Model file for the job. Use its own axes, mm. A direction names the side the tool comes from. Give positions to 0.01 mm unless a question says otherwise; leave off trailing zeros. Loops run counter-clockwise (first coordinate to the right, second up) from the corner with the lowest first, then second, coordinate; pieces in that order, holes last. Notation, with made-up numbers: (69.5, -7.5) -> (89.5, -7.5) arc R31 cw to (89.5, 25.5) -> close; hole circle Ø9 at (37.25, 19). An arc over 180 degrees is marked (long way). Use CSV: the item, a comma, the result in double quotes. Start each with the question number.
(1) Cut at B-B on y = 0.5. Write the cut outline in (x, z), then the cut area to 3 significant figures.
(2) Pull direction Y, two halves, no side cores. Call faces 6 (the cylindrical face through (4, 24, 0)), 7 (the cylindrical face through (-8.028, -9.157, -0.111)), 8 (the cylindrical face through (-0.084, 12.926, -0.238)), 9 (the flat face through (-3, 8, -10)): pulls with the +Y half, pulls with the -Y half, needs draft (parallel to the pull), parting line crosses it, or undercut.
(3) Flat gauge pins, fed straight in: pin 1 (1.3 mm diameter, centred on y = 14, z = 0, fed in from -X); pin 2 (1.5 mm diameter, centred on y = 8, z = 5, fed in from +X); pin 3 (6 mm diameter, centred on y = 14.5, z = 0, fed in from -X); pin 4 (1.5 mm diameter, centred on x = 4, z = 6, fed in from +Y). Where does each tip first touch, or does it go through?
(4) 3-axis set-ups, long thin cutter, end or side, ignore diameter. For faces 1 (the cylindrical face through (-8.859, -3.098, -8.797)), 2 (the flat face through (-2, 7, 5)), 3 (the flat face through (-8, 4, 0)), 4 (the flat face through (8, 4, 0)), 5 (the cylindrical face through (0.3, 2, 5.6)): which of +Z, -Z, +X, -X, +Y, -Y reach the whole face in a straight line?
(5) Cut at D-D on x = 6.5. Write the cut outline in (y, z), then the cut area to 3 significant figures.
(6) Drill centre lines: probe 1 along Y at (x, z) = (-5, 0); probe 2 along X at (y, z) = (3.15, -6); probe 3 along X at (y, z) = (5, 6.25). Where is each one in solid material? Low to high.
(7) Cut at C-C on x = -2.75. Write the cut outline in (y, z), then the cut area to 3 significant figures.
from build123d import *

# Parameters (mm, degrees)
SKETCH1_W           = 20
SKETCH1_H           = 20
BOSS_EXTRUDE1_DEPTH = 4
SKETCH4_W           = 4
SKETCH4_H           = 20
BOSS_EXTRUDE2_DEPTH = 10
BOSS_EXTRUDE3_DEPTH = 4
BOSS_EXTRUDE4_START = -4
BOSS_EXTRUDE4_DEPTH = 4
SKETCH7_R           = 0.85
CUT_EXTRUDE1_DEPTH  = 31
FILLET1_R           = 4
SKETCH8_W           = 4
SKETCH8_H           = 20
BOSS_EXTRUDE5_DEPTH = 10
SKETCH9_R           = 10
BOSS_EXTRUDE6_DEPTH = 4
BOSS_EXTRUDE7_START = -4
SKETCH10_R          = 10
BOSS_EXTRUDE7_DEPTH = 4
SKETCH12_R          = 1.1
CUT_EXTRUDE2_DEPTH  = 31.528675045
SKETCH13_R          = 6
BOSS_EXTRUDE8_DEPTH = 4
SKETCH14_R          = 1.1
CUT_EXTRUDE3_DEPTH  = 4
FILLET2_R           = 2
CUT_EXTRUDE4_REACH  = 29.857
SKETCH16_R          = 0.5


with BuildPart() as part:
    # Sketch1 → Boss-Extrude1 (new body)
    with BuildSketch(Plane(origin=(0, 0, 0), x_dir=(1, 0, 0), z_dir=(0, 1, 0))):
        Rectangle(SKETCH1_W, SKETCH1_H)
    extrude(amount=BOSS_EXTRUDE1_DEPTH)

    # Sketch4 → Boss-Extrude2 (add)
    with BuildSketch(Plane.XZ):
        with Locations((-8, 0)):
            Rectangle(SKETCH4_W, SKETCH4_H)
        with Locations((8, 0)):
            Rectangle(SKETCH4_W, SKETCH4_H)
    extrude(amount=BOSS_EXTRUDE2_DEPTH)

    # Sketch5 → Boss-Extrude3 (add)
    with BuildSketch(Plane.ZY.offset(10)):
        with BuildLine():
            Line((0, -20), (10, -20))
            Line((10, -20), (10, -10))
            ThreePointArc((10, -10), (-7.071067812, -2.928932188), (0, -20))
        make_face()
    extrude(amount=-BOSS_EXTRUDE3_DEPTH)

    # Sketch6 → Boss-Extrude4 (add)
    with BuildSketch(Plane(origin=(10, 0, 0), x_dir=(0, 0, -1), z_dir=(1, 0, 0)).offset(BOSS_EXTRUDE4_START)):
        with BuildLine():
            Line((0, -20), (-10, -20))
            Line((-10, -20), (-10, -10))
            ThreePointArc((-10, -10), (7.071067812, -2.928932188), (0, -20))
        make_face()
    extrude(amount=BOSS_EXTRUDE4_DEPTH)

    # Sketch7 → Cut-Extrude1 (cut, through all)
    with BuildSketch(Plane.ZY.offset(10)):
        with Locations((0, -10)):
            Circle(SKETCH7_R)
    extrude(amount=-CUT_EXTRUDE1_DEPTH, mode=Mode.SUBTRACT)

    # Fillet1
    fillet1_edges = [part.edges().sort_by_distance(p)[0] for p in [
        (-10, -8, 10),
        (-10, -17.071067812, -7.071067812),
        (10, -8, 10),
        (10, -17.071067812, -7.071067812),
        (-10, -3, -10),
        (10, -3, -10),
        (10, -20, 5),
        (-10, -20, 5),
    ]]
    fillet(fillet1_edges, radius=FILLET1_R - 0.0001)  # a hair under: the kernel refuses the full size

    # Sketch8 → Boss-Extrude5 (add)
    with BuildSketch(Plane(origin=(0, 4, 0), x_dir=(1, 0, 0), z_dir=(0, 1, 0))):
        with Locations((4, 0)):
            Rectangle(SKETCH8_W, SKETCH8_H)
        with Locations((-4, 0)):
            Rectangle(SKETCH8_W, SKETCH8_H)
    extrude(amount=BOSS_EXTRUDE5_DEPTH)

    # Sketch9 → Boss-Extrude6 (add)
    with BuildSketch(Plane(origin=(6, 0, 0), x_dir=(0, 0, -1), z_dir=(1, 0, 0))):
        with Locations((0, 14)):
            Circle(SKETCH9_R)
    extrude(amount=-BOSS_EXTRUDE6_DEPTH)

    # Sketch10 → Boss-Extrude7 (add)
    with BuildSketch(Plane.ZY.offset(6).offset(BOSS_EXTRUDE7_START)):
        with Locations((0, 14)):
            Circle(SKETCH10_R)
    extrude(amount=BOSS_EXTRUDE7_DEPTH)

    # Sketch12 → Cut-Extrude2 (cut, through all)
    with BuildSketch(Plane.ZY.offset(6)):
        with Locations((0, 14)):
            Circle(SKETCH12_R)
    extrude(amount=-CUT_EXTRUDE2_DEPTH, mode=Mode.SUBTRACT)

    # Sketch13 → Boss-Extrude8 (add)
    with BuildSketch(Plane(origin=(-2, 0, 0), x_dir=(0, 0, -1), z_dir=(1, 0, 0))):
        with Locations(Location((0, 14, 0), (0, 0, 180))):
            Circle(SKETCH13_R)
    extrude(amount=BOSS_EXTRUDE8_DEPTH)

    # Sketch14 → Cut-Extrude3 (cut)
    with BuildSketch(Plane(origin=(-2, 0, 0), x_dir=(0, 0, -1), z_dir=(1, 0, 0))):
        with Locations(Location((0, 14, 0), (0, 0, 180))):
            Circle(SKETCH14_R)
    extrude(amount=CUT_EXTRUDE3_DEPTH, mode=Mode.SUBTRACT)

    # Fillet2
    fillet2_edges = [part.edges().sort_by_distance(p)[0] for p in [
        (-2, 14, -6),
        (2, 14, -6),
    ]]
    fillet(fillet2_edges, radius=FILLET2_R - 0.0001)  # a hair under: the kernel refuses the full size

    # Sketch16 → Cut-Extrude4 (cut, up to next)
    with BuildSketch(Plane.XZ, mode=Mode.PRIVATE) as cut_extrude4_sk1:
        with Locations(Location((0, -6, 0), (0, 0, 270))):
            Circle(SKETCH16_R)
    cut_extrude4_tool1 = extrude(cut_extrude4_sk1.sketch, amount=-CUT_EXTRUDE4_REACH, mode=Mode.PRIVATE) & part.part
    # Sketch16 → Cut-Extrude4 (cut, up to next)
    with BuildSketch(Plane.XZ, mode=Mode.PRIVATE) as cut_extrude4_sk2:
        with Locations(Location((0, 6, 0), (0, 0, 90))):
            Circle(SKETCH16_R)
    cut_extrude4_tool2 = extrude(cut_extrude4_sk2.sketch, amount=-CUT_EXTRUDE4_REACH, mode=Mode.PRIVATE) & part.part
    add(cut_extrude4_tool1.solids().sort_by_distance((0, 0, -6))[0], mode=Mode.SUBTRACT)
    add(cut_extrude4_tool2.solids().sort_by_distance((0, 0, 6))[0], mode=Mode.SUBTRACT)


solid = part.part
Check result:
1,outline,"(-10, -6) arc R4 ccw to (-6, -10) -> (6, -10) arc R4 ccw to (10, -6) -> (10, 6) arc R4 ccw to (6, 10) -> (-6, 10) arc R4 ccw to (-10, 6) -> close; hole circle Ø1 at (0, -6); hole circle Ø1 at (0, 6)"
1,area,"385 mm²"
2,face 6,"pulls with the +Y half"
2,face 7,"undercut"
2,face 8,"undercut"
2,face 9,"needs draft"
3,pin 1,"through"
3,pin 2,"x = 6"
3,pin 3,"x = -6"
3,pin 4,"y = 22.51"
4,face 1,"-Z, -X, +Y, -Y"
4,face 2,"none"
4,face 3,"+Z, -Z, -X, +Y"
4,face 4,"+Z, -Z, +X, +Y"
4,face 5,"-Y"
5,outline,"(-19.97, 0) arc R9.97 ccw to (-10, -9.97) -> (4, -9.97) -> (4, 9.97) -> (-19.97, 9.97) -> close; hole circle Ø1.7 at (-10, 0)"
5,area,"454 mm²"
6,probe 1,"0 to 12.9, 15.1 to 24"
6,probe 2,"-10 to -0.5, 0.5 to 10"
6,probe 3,"-6 to -2, 2 to 6"
7,outline,"(0, -10) -> (14, -10) arc R10 ccw to (14, 10) -> (0, 10) -> close; hole circle Ø2.2 at (14, 0)"
7,area,"433 mm²"
